```python
from build123d import *

# Parameters (mm, degrees)
F0_W        = 9
F0_H        = 35
F0_R        = 1.6
F1_DEPTH    = 3.2
F2_T1_DEPTH = 28.2


# Not quite as in the source:
# - a fillet or chamfer that OpenCascade refuses, or shapes differently, is made with other operations: its cross-section is extruded or revolved along the edge and cut away or added


with BuildPart() as f1:
    # F0 (on Front) → F1 (new body)
    with BuildSketch(Plane.XZ):
        with Locations((-14.7368423641, 13.5)):
            Rectangle(F0_W, F0_H)
        with Locations((-14.7368423641, 0)):
            Circle(F0_R, mode=Mode.SUBTRACT)
        with Locations((-14.7368423641, 25.4)):
            Circle(F0_R, mode=Mode.SUBTRACT)
    extrude(amount=F1_DEPTH)

    # F2: fillet of radius 5 on 4 edges, made by hand

    # F2_s2 → F2_t1 (cut)
    with BuildSketch(Plane.XZ.offset(-12.5)):
        with BuildLine():
            ThreePointArc((-10.2368423641, 26), (-11.7013084581, 29.5355339059), (-15.2368423641, 31))
            Line((-15.2368423641, 31), (-10.2368423641, 31))
            Line((-10.2368423641, 31), (-10.2368423641, 26))
        make_face()
        with BuildLine():
            ThreePointArc((-14.2368423641, 31), (-17.77237627, 29.5355339059), (-19.2368423641, 26))
            Line((-19.2368423641, 26), (-19.2368423641, 31))
            Line((-19.2368423641, 31), (-14.2368423641, 31))
        make_face()
        with BuildLine():
            ThreePointArc((-10.2368423641, 1), (-11.7013084581, -2.5355339059), (-15.2368423641, -4))
            Line((-15.2368423641, -4), (-10.2368423641, -4))
            Line((-10.2368423641, -4), (-10.2368423641, 1))
        make_face()
        with BuildLine():
            ThreePointArc((-19.2368423641, 1), (-17.77237627, -2.5355339059), (-14.2368423641, -4))
            Line((-14.2368423641, -4), (-19.2368423641, -4))
            Line((-19.2368423641, -4), (-19.2368423641, 1))
        make_face()
    extrude(amount=F2_T1_DEPTH, mode=Mode.SUBTRACT)


solid = f1.part
```
The listing builds one solid part. Answer for the finished solid, in the listing's coordinates (mm). Give positions to 0.01 mm unless a question says otherwise; leave off trailing zeros. Loops run counter-clockwise (first coordinate to the right, second up) from the corner with the lowest first, then second, coordinate; pieces in that order, holes last. Notation, with made-up numbers: (27.25, -28.5) - (72.25, -28.5) arc R33 cw to (72.25, 6.5) - close; hole circle Ø10 at (88.5, 56). An arc over 180 degrees is marked (long way). Answer as CSV lines item,"result". Start each with the question number.
Item 1: A cutting plane is placed at B-B on y = -2.6. Determine the outline of the cut face in (x, z), then the cut area to 3 significant figures.
Item 2: A cutting plane is placed at A-A on z = 25.4. Determine the outline of the cut face in (x, y), then the cut area to 3 significant figures.
Item 3: The mould has two halves that part along Z. Classify faces 1 (the face through (-17.979, -1.578, -2.316)), 2 (the face through (-10.237, -2, 13)), 3 (the face through (-13.21, -1.58, 0.48)): +Z half, -Z half, draft (parallel to the pull), parting line (faces both ways), or undercut.
Item 4: Find the intervals of material crossed by line 1 (Z direction, x = -13.75, y = -0.05); line 2 (Z direction, x = -15.5, y = -0.6); line 3 (Z direction, x = -12, y = -0.8), in increasing order. Write a range as from..to.
Item 5: A cutting plane is placed at D-D on z = 0. Determine the outline of the cut face in (x, y).
Item 6: This flat-tipped pin is pushed along its axis until it touches: pin 1 (2.5 mm diameter, centred on x = -14.74, z = 0, fed in from +Y). Where does it stop, or does it pass through?
Item 7: A cutting plane is placed at C-C on x = -15.5. Determine the outline of the cut face in (y, z), then the cut area to 3 significant figures.
Found:
1,outline,"(-19.24, 1) arc R5 ccw to (-14.74, -3.97) arc R5 ccw to (-10.24, 1) - (-10.24, 26) arc R5 ccw to (-14.74, 30.97) arc R5 ccw to (-19.24, 26) - close; hole circle Ø3.2 at (-14.74, 0); hole circle Ø3.2 at (-14.74, 25.4)"
1,area,"277 mm^2"
2,outline,"(-19.24, -3.2) - (-16.34, -3.2) - (-16.34, 0) - (-19.24, 0) - close; (-13.14, -3.2) - (-10.24, -3.2) - (-10.24, 0) - (-13.14, 0) - close"
2,area,"18.6 mm^2"
3,face 1,"-Z half"
3,face 2,"draft"
3,face 3,"undercut"
4,line 1,"z = -3.77..-1.26, 1.26..24.14, 26.66..30.77"
4,line 2,"z = -3.84..-1.41, 1.41..23.99, 26.81..30.84"
4,line 3,"z = -2.81..29.81"
5,outline,"(-19.14, -3.2) - (-16.34, -3.2) - (-16.34, 0) - (-19.14, 0) - close; (-13.14, -3.2) - (-10.34, -3.2) - (-10.34, 0) - (-13.14, 0) - close"
6,pin 1,"passes through"
7,outline,"(-3.2, -3.84) - (0, -3.84) - (0, -1.41) - (-3.2, -1.41) - close; (-3.2, 1.41) - (0, 1.41) - (0, 23.99) - (-3.2, 23.99) - close; (-3.2, 26.81) - (0, 26.81) - (0, 30.84) - (-3.2, 30.84) - close"
7,area,"93.0 mm^2"
